```python
from build123d import *

# Parameters (mm, degrees)
ESBO_O1_W                                    = 31
ESBO_O1_H                                    = 49
RESSALTO_EXTRUS_O1_DEPTH                     = 9.5
REBAIXO_PARA_PARAFUSO_COM_CABE_A_RED_2_COUNT = 2
REBAIXO_PARA_PARAFUSO_COM_CABE_A_RED_2_PITCH = 35
REBAIXO_PARA_PARAFUSO_COM_CABE_A_RED_3_COUNT = 2
REBAIXO_PARA_PARAFUSO_COM_CABE_A_RED_3_PITCH = 49.497474683
REBAIXO_PARA_PARAFUSO_COM_CABE_A_RED_4_COUNT = 2
REBAIXO_PARA_PARAFUSO_COM_CABE_A_RED_4_PITCH = 35
ESBO_O8_R                                    = 19.9
RESSALTO_EXTRUS_O2_DEPTH                     = 5.5
ESBO_O5_R                                    = 16.5
CORTE_EXTRUS_O1_DEPTH                        = 92.787798753
CHANFRO1_SIZE                                = 0.5


with BuildPart() as part:
    # Esboço1 → Ressalto-extrusão1 (new body)
    with BuildSketch(Plane(origin=(0, 0, 0), x_dir=(0, 0, -1), z_dir=(1, 0, 0))):
        Polygon((16.5, 66), (0, 49), (31, 49), (31, 66), align=None)
        Polygon((31, 66), (31, 49), (62, 49), (45.5, 66), align=None)
        with Locations((15.5, 24.5)):
            Rectangle(ESBO_O1_W, ESBO_O1_H)
        with Locations((46.5, 24.5)):
            Rectangle(ESBO_O1_W, ESBO_O1_H)
    extrude(amount=-RESSALTO_EXTRUS_O1_DEPTH)

    # Esboço4 → Rebaixo para parafuso com cabeça redonda de M61 (revolve, cut)
    with BuildSketch(Plane(origin=(0, 52, -13.5), x_dir=(0, 0, -1), z_dir=(0, 1, 0))):
        Polygon((0, 0), (0, 9.5), (3.3, 9.5), (3.3, 5.5), (5.5, 5.5), (5.5, 0.025), (5.525, 0), align=None)
    rebaixo_para_parafuso_com_cabe_a_redonda = revolve(axis=Axis((6.35, 52, -13.5), (-1, 0, 0)), mode=Mode.SUBTRACT)

    # Rebaixo para parafuso com cabe_a red 2: Rebaixo para parafuso com cabeça redonda de M61 ×2
    with Locations(*[(0, 0, -i * REBAIXO_PARA_PARAFUSO_COM_CABE_A_RED_2_PITCH) for i in range(1, REBAIXO_PARA_PARAFUSO_COM_CABE_A_RED_2_COUNT)]):
        add(rebaixo_para_parafuso_com_cabe_a_redonda, mode=Mode.SUBTRACT)

    # Rebaixo para parafuso com cabe_a red 3: Rebaixo para parafuso com cabeça redonda de M61 ×2
    with Locations(*[Vector(0, -0.7071067811865477, -0.7071067811865475) * (i * REBAIXO_PARA_PARAFUSO_COM_CABE_A_RED_3_PITCH) for i in range(1, REBAIXO_PARA_PARAFUSO_COM_CABE_A_RED_3_COUNT)]):
        add(rebaixo_para_parafuso_com_cabe_a_redonda, mode=Mode.SUBTRACT)

    # Rebaixo para parafuso com cabe_a red 4: Rebaixo para parafuso com cabeça redonda de M61 ×2
    with Locations(*[(0, -i * REBAIXO_PARA_PARAFUSO_COM_CABE_A_RED_4_PITCH, 0) for i in range(1, REBAIXO_PARA_PARAFUSO_COM_CABE_A_RED_4_COUNT)]):
        add(rebaixo_para_parafuso_com_cabe_a_redonda, mode=Mode.SUBTRACT)

    # Esboço8 → Ressalto-extrusão2 (add)
    with BuildSketch(Plane.ZY.offset(9.5)):
        with Locations(Location((-31, 34.5, 0), (0, 0, 180))):
            Circle(ESBO_O8_R)
    extrude(amount=RESSALTO_EXTRUS_O2_DEPTH)

    # Esboço5 → Corte-extrusão1 (cut, through all)
    with BuildSketch(Plane(origin=(0, 0, 0), x_dir=(0, 0, -1), z_dir=(1, 0, 0))):
        with Locations((31, 34.5)):
            Circle(ESBO_O5_R)
    extrude(amount=-CORTE_EXTRUS_O1_DEPTH, mode=Mode.SUBTRACT)

    # Chanfro1
    chanfro1_edges = [part.edges().sort_by_distance(p)[0] for p in [
        (0, 34.5, -14.5),
    ]]
    chamfer(chanfro1_edges, length=CHANFRO1_SIZE)


solid = part.part
```
Source: CAD feature listing. Evaluate the final solid. Frame: model axes, mm. A direction names the side the tool comes from. Give positions to 0.01 mm unless a question says otherwise; leave off trailing zeros. Loops run counter-clockwise (first coordinate to the right, second up) from the corner with the lowest first, then second, coordinate; pieces in that order, holes last. Notation, with made-up numbers: (49, -33) -> (102, -33) arc R13 ccw to (102, -23) -> close; hole circle Ø8 at (-24.5, 24.5). An arc over 180 degrees is marked (long way). Use a Markdown table: item, result. Add a question column.
(1) Section query C-C (x = -12.75). Output: boundary loops of the cut face in (y, z).
(2) Access query for faces 4 (the face through (-5.5, 17, -10)), 5 (the face through (-9.5, 19, -17)), 6 (the face through (0, 18.8, -23.7)). Directions: +Z, -Z, +X, -X, +Y, -Y. A direction counts if a zero-diameter tool reaches every point of the face in a straight line with its end or side. Return the directions, or none.
(3) Section query A-A (y = 34.5). Output: boundary loops of the cut face in (x, z), then the cut area to 3 significant figures.
(4) Ray query, line 1 (Z direction, x = -1.55, y = 52); line 2 (Y direction, x = -2.95, z = -13.5); line 3 (Y direction, x = -7.3, z = -13.5). Return the intervals inside material, ascending.
(5) First-contact query: pin 1 Ø5.5 at (y, z) = (52, -48.5) entering from -X; pin 2 Ø8.5 at (y, z) = (17, -48.5) entering from +X. Flat tips, straight axial feed; report the tip coordinate or a pass-through.
(6) Pull-direction query (Y, two-part tool) for faces 1 (the face through (-5, 24, -62)), 2 (the face through (-4.684, 57.381, -53.866)), 3 (the face through (-5.5, 21, -49)); classes: +Y half, -Y half, draft (parallel to the pull), parting line (faces both ways), or undercut.
(7) Section query B-B (z = -31). Output: boundary loops of the cut face in (x, y).
(8) Section query D-D (z = -6.5). Output: boundary loops of the cut face in (x, y).
Checked values:
| question | item | result |
|---|---|---|
| 1 | outline | circle Ø39.8 at (34.5, -31); hole circle Ø33 at (34.5, -31) |
| 2 | face 4 | +X |
| 2 | face 5 | -X |
| 2 | face 6 | +Z, -Z, +X, +Y, -Y |
| 3 | outline | (-15, -50.9) -> (-9.5, -50.9) -> (-9.5, -62) -> (0, -62) -> (0, -48) -> (-0.5, -47.5) -> (-15, -47.5) -> close; (-15, -14.5) -> (-0.5, -14.5) -> (0, -14) -> (0, 0) -> (-9.5, 0) -> (-9.5, -11.1) -> (-15, -11.1) -> close |
| 3 | area | 313 mm^2 |
| 4 | line 1 | -59.09 to -54, -43 to -19, -8 to -2.91 |
| 4 | line 2 | 0 to 11.5, 22.5 to 46.5, 57.5 to 62.91 |
| 4 | line 3 | 0 to 13.7, 20.3 to 48.7, 55.3 to 62.91 |
| 5 | pin 1 | through |
| 5 | pin 2 | x = -5.5 |
| 6 | face 1 | draft |
| 6 | face 2 | +Y half |
| 6 | face 3 | undercut |
| 7 | outline | (-15, 14.6) -> (-9.5, 14.6) -> (-9.5, 0) -> (0, 0) -> (0, 17.5) -> (-0.5, 18) -> (-15, 18) -> close; (-15, 51) -> (-0.5, 51) -> (0, 51.5) -> (0, 66) -> (-9.5, 66) -> (-9.5, 54.4) -> (-15, 54.4) -> close |
| 8 | outline | (-9.5, 0) -> (0, 0) -> (0, 55.7) -> (-9.5, 55.7) -> close |
